Work out the finished part from the listing and answer in its coordinate system (mm). Face numbers are marked on the shaded views. A direction names the side the tool comes from. Give positions to 0.01 mm unless a question says otherwise; leave off trailing zeros. Loops run counter-clockwise (first coordinate to the right, second up) from the corner with the lowest first, then second, coordinate; pieces in that order, holes last. Notation, with made-up numbers: M 27,66 L 42,66 A19 cw 42,100 Z; hole C 38,50.5 d9. An arc over 180 degrees is marked long. Write item = value, one per line. Start each with the question number.
1. The mould has two halves that part along Z. Classify the marked faces 3, 4, 5 and 6: released by +Z, released by -Z, zero draft, split by the parting line, or undercut.
2. Section B-B on y = -33.5 is taken. Determine the outline of the cut face in (x, z).
3. Flat-ended cylindrical pins translate along their axes: pin 1 Ø1.6 at (y, z) = (-1.5, 14.5) entering from +X; pin 2 Ø3 at (x, z) = (-32, -18) entering from -Y; pin 3 Ø0.6 at (x, y) = (-13.5, -1.5) entering from +Z. Find the tip coordinate at first contact, or state that the pin passes through.
4. Section D-D on z = -1 is taken. Determine the outline of the cut face in (x, y).
5. For the marked faces 1 and 2, determine the directions among +Z, -Z, +X, -X, +Y, -Y from which every point of the face is accessible in a straight line to the end or side of a thin tool.
6. Consider L1, parallel to Z at x = -38.5, y = -8.5; L2, parallel to X at y = -30.5, z = -27; L3, parallel to Y at x = -40, z = 19. Determine where each line is inside the solid, lowest interval first. Write a range as [from, to].
7. Section A-A on z = -15 is taken. Determine the outline of the cut face in (x, y), plus the area to 3 significant figures.
8. Section C-C on y = -19 is taken. Determine the outline of the cut face in (x, z), plus the area to 3 significant figures.
```python
from build123d import *

# Parameters (mm, degrees)
SKETCH1_W           = 105
SKETCH1_H           = 57
BOSS_EXTRUDE1_DEPTH = 2
SKETCH2_W           = 109
SKETCH2_H           = 61
SKETCH2_W_2         = 105
SKETCH2_H_2         = 57
BOSS_EXTRUDE2_DEPTH = 40
SKETCH3_W           = 13
SKETCH3_H           = 14
SKETCH3_W_2         = 10
CUT_EXTRUDE1_DEPTH  = 2
SKETCH4_W           = 3
SKETCH4_H           = 3
CUT_EXTRUDE2_DEPTH  = 2
LPATTERN1_COUNT     = 6
LPATTERN1_PITCH     = 10
SKETCH5_W           = 3
SKETCH5_H           = 3
CUT_EXTRUDE3_DEPTH  = 2
LPATTERN2_COUNT     = 6
LPATTERN2_PITCH     = 10
SKETCH6_W           = 3
SKETCH6_H           = 3
CUT_EXTRUDE4_DEPTH  = 2
SKETCH7_W           = 3
SKETCH7_H           = 3
CUT_EXTRUDE5_DEPTH  = 2
FILLET2_R           = 2.5


with BuildPart() as part:
    # Sketch1 → Boss-Extrude1 (new body)
    with BuildSketch(Plane(origin=(0, 0, 0), x_dir=(1, 0, 0), z_dir=(0, 1, 0))):
        Rectangle(SKETCH1_W, SKETCH1_H)
    extrude(amount=-BOSS_EXTRUDE1_DEPTH)

    # Sketch2 → Boss-Extrude2 (add)
    with BuildSketch(Plane(origin=(0, 0, 0), x_dir=(1, 0, 0), z_dir=(0, 1, 0))):
        Rectangle(SKETCH2_W, SKETCH2_H)
        Rectangle(SKETCH2_W_2, SKETCH2_H_2, mode=Mode.SUBTRACT)
    extrude(amount=-BOSS_EXTRUDE2_DEPTH)

    # Sketch3 → Cut-Extrude1 (cut)
    with BuildSketch(Plane.ZY.offset(54.5)):
        with Locations((-15, -33)):
            Rectangle(SKETCH3_W, SKETCH3_H)
        with Locations((18.5, -33)):
            Rectangle(SKETCH3_W_2, SKETCH3_H)
    extrude(amount=-CUT_EXTRUDE1_DEPTH, mode=Mode.SUBTRACT)

    # Sketch4 → Cut-Extrude2 (cut)
    with BuildSketch(Plane(origin=(0, 0, 0), x_dir=(1, 0, 0), z_dir=(0, 1, 0))):
        with Locations((-23, -14)):
            Rectangle(SKETCH4_W, SKETCH4_H)
    cut_extrude2 = extrude(amount=-CUT_EXTRUDE2_DEPTH, mode=Mode.SUBTRACT)

    # LPattern1: Cut-Extrude2 ×6
    with Locations(*[(i * LPATTERN1_PITCH, 0, 0) for i in range(1, LPATTERN1_COUNT)]):
        add(cut_extrude2, mode=Mode.SUBTRACT)

    # Sketch5 → Cut-Extrude3 (cut)
    with BuildSketch(Plane(origin=(0, 0, 0), x_dir=(1, 0, 0), z_dir=(0, 1, 0))):
        with Locations((-18, 7)):
            Rectangle(SKETCH5_W, SKETCH5_H)
    cut_extrude3 = extrude(amount=-CUT_EXTRUDE3_DEPTH, mode=Mode.SUBTRACT)

    # LPattern2: Cut-Extrude3 ×6
    with Locations(*[(i * LPATTERN2_PITCH, 0, 0) for i in range(1, LPATTERN2_COUNT)]):
        add(cut_extrude3, mode=Mode.SUBTRACT)

    # Sketch6 → Cut-Extrude4 (cut)
    with BuildSketch(Plane(origin=(0, 0, 0), x_dir=(1, 0, 0), z_dir=(0, 1, 0))):
        with Locations((-14, 15)):
            Rectangle(SKETCH6_W, SKETCH6_H)
        with Locations((-3, 12.331798483)):
            Rectangle(SKETCH6_W, SKETCH6_H)
    extrude(amount=-CUT_EXTRUDE4_DEPTH, mode=Mode.SUBTRACT)

    # Sketch7 → Cut-Extrude5 (cut)
    with BuildSketch(Plane(origin=(0, 0, 0), x_dir=(1, 0, 0), z_dir=(0, 1, 0))):
        with Locations((-33, -9)):
            Rectangle(SKETCH7_W, SKETCH7_H)
        with Locations((26, 12)):
            Rectangle(SKETCH7_W, SKETCH7_H)
        with Locations((31, -19)):
            Rectangle(SKETCH7_W, SKETCH7_H)
    extrude(amount=-CUT_EXTRUDE5_DEPTH, mode=Mode.SUBTRACT)

    # Fillet2
    fillet2_edges = [part.edges().sort_by_distance(p)[0] for p in [
        (-54.5, 0, 0),
        (0, 0, 30.5),
        (54.5, 0, 0),
        (0, 0, -30.5),
    ]]
    fillet(fillet2_edges, radius=FILLET2_R)


solid = part.part
```
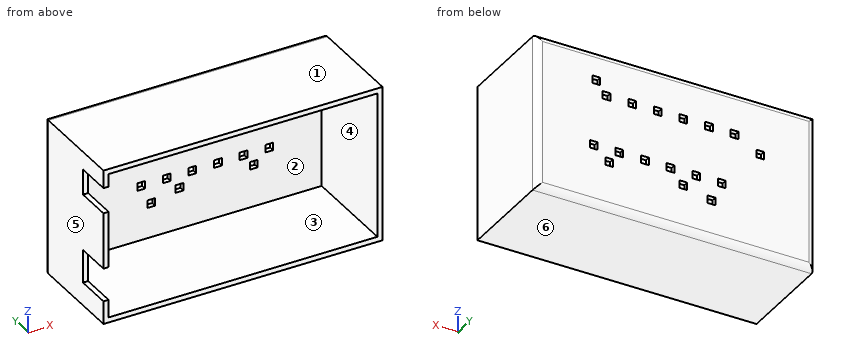
Verdict:
q1.face_3 = undercut
q1.face_4 = undercut
q1.face_5 = zero draft
q1.face_6 = released by -Z
q2.outline = M -54.5,-30.5 L 54.5,-30.5 L 54.5,30.5 L -54.5,30.5 L -54.5,23.5 L -52.5,23.5 L -52.5,28.5 L 52.5,28.5 L 52.5,-28.5 L -52.5,-28.5 L -52.5,-21.5 L -54.5,-21.5 Z; M -54.5,-8.5 L -52.5,-8.5 L -52.5,13.5 L -54.5,13.5 Z
q3.pin_1 = 54.49
q3.pin_2 = -2
q3.pin_3 = 30.4
q4.outline = M -54.5,-40 L -52.5,-40 L -52.5,-2 L 52.5,-2 L 52.5,-40 L 54.5,-40 L 54.5,-2.5 A2.5 ccw 52,0 L -52,0 A2.5 ccw -54.5,-2.5 Z
q5.face_1 = +Z, +X, -X, +Y, -Y
q5.face_2 = -Y
q6.L1 = [-30.5, -28.5], [28.5, 30.5]
q6.L2 = [-54.5, -52.5], [52.5, 54.5]
q6.L3 = [-2, 0]
q7.outline = M -54.5,-26 L -52.5,-26 L -52.5,-2 L -15.5,-2 L -15.5,0 L -52,0 A2.5 ccw -54.5,-2.5 Z; M -12.5,-2 L 52.5,-2 L 52.5,-40 L 54.5,-40 L 54.5,-2.5 A2.5 ccw 52,0 L -12.5,0 Z
q7.area = 333 mm2
q8.outline = M -54.5,-30.5 L 54.5,-30.5 L 54.5,30.5 L -54.5,30.5 Z; hole M -52.5,-28.5 L 52.5,-28.5 L 52.5,28.5 L -52.5,28.5 Z
q8.area = 664 mm2
